```python
from build123d import *

# Parameters (mm, degrees)
CIRPATTERN1_COUNT = 8


with BuildPart() as part:
    # Sketch1 → Revolve2 (revolve)
    with BuildSketch(Plane.XY, mode=Mode.PRIVATE) as revolve2_sk:
        with BuildLine():
            Line((71.638455479, 109.927347077), (76.2, 109.927347077))
            Line((76.2, 109.927347077), (76.2, -212.12767375))
            Line((76.2, -212.12767375), (53.792460136, -212.12767375))
            Line((53.792460136, -212.12767375), (53.792460136, -59.72767375))
            add(Edge.make_bspline(
                [(53.792460136, -59.72767375), (53.792458904, -59.65714368), (53.79192976, -59.515566627), (53.789553906, -59.18172514), (53.783229304, -58.904956016), (53.773743812, -58.532728011), (53.761100911, -58.212998146), (53.741350078, -57.781754967), (53.711337732, -57.281120424), (53.667125562, -56.68815869), (53.588220883, -55.848640892), (53.488359283, -55.008326387), (53.367608198, -54.172595959), (53.197743223, -53.17258577), (53.002996576, -52.177603354), (52.777307499, -51.188699619), (52.520946592, -50.207649576), (52.240221697, -49.233238281), (51.935281085, -48.266129768), (51.544470164, -47.149295616), (51.050452679, -45.89056896), (50.509666057, -44.651129364), (49.922993218, -43.432862093), (49.291052508, -42.237253813), (48.615057493, -41.066315461), (47.895407771, -39.921133247), (47.134034376, -38.804236838), (46.430801288, -37.851612392), (45.804470156, -37.055832736), (45.263749892, -36.403541902), (44.826059154, -35.894408258), (44.42570839, -35.447153287), (44.092389699, -35.084791818), (43.784856817, -34.760500788), (43.585004597, -34.55171009), (43.35532426, -34.318676929), (43.254715338, -34.217322698), (43.20484319, -34.167450311)],
                knots=[0.082637729, 0.082637729, 0.082637729, 0.082637729, 0.082637729, 0.092574926, 0.102512123, 0.11244932, 0.122386517, 0.132323714, 0.142260911, 0.162135305, 0.182009699, 0.201884093, 0.24163288, 0.261507274, 0.281381668, 0.321130456, 0.360879243, 0.380753637, 0.400628031, 0.440376819, 0.480125606, 0.519874394, 0.559623181, 0.599371969, 0.639120757, 0.678869544, 0.718618332, 0.75836712, 0.798115907, 0.817990301, 0.837864695, 0.857739089, 0.877613483, 0.88755068, 0.897487877, 0.907425074, 0.91736227, 0.91736227, 0.91736227, 0.91736227, 0.91736227], degree=4))
            Line((43.20484319, -34.167450311), (34.597214993, -25.559822115))
            add(Edge.make_bspline(
                [(24.01, 0), (24.010001231, -0.070528647), (24.010530378, -0.21358419), (24.012906064, -0.543182916), (24.019230459, -0.824160397), (24.028715581, -1.194822072), (24.041357874, -1.513435058), (24.057158099, -1.861939603), (24.076113358, -2.193706872), (24.103750973, -2.6180694), (24.143219181, -3.122033947), (24.214231843, -3.879978675), (24.334058816, -4.886450388), (24.510418185, -6.05671076), (24.761817377, -7.385166415), (25.062727461, -8.703574514), (25.412702774, -10.009637208), (25.811293137, -11.301819596), (26.257877549, -12.578099334), (26.751935483, -13.836887483), (27.292605285, -15.076197128), (27.879411553, -16.294609793), (28.511071567, -17.489938793), (29.187464568, -18.661287756), (29.906377277, -19.805743395), (30.668954178, -20.923860073), (31.370099373, -21.874411759), (31.999668305, -22.673445479), (32.535060601, -23.320422136), (32.983187953, -23.840005015), (33.419382213, -24.329816244), (33.846758309, -24.788484388), (34.156490828, -25.113868308), (34.447792147, -25.409649045), (34.547344615, -25.50994993), (34.597214993, -25.559822115)],
                knots=[0.082637729, 0.082637729, 0.082637729, 0.082637729, 0.082637729, 0.092574926, 0.102512123, 0.11244932, 0.122386517, 0.132323714, 0.142260911, 0.152198108, 0.162135305, 0.182009699, 0.201884093, 0.24163288, 0.281381668, 0.321130456, 0.360879243, 0.400628031, 0.440376819, 0.480125606, 0.519874394, 0.559623181, 0.599371969, 0.639120757, 0.678869544, 0.718618332, 0.75836712, 0.798115907, 0.817990301, 0.837864695, 0.857739089, 0.877613483, 0.897487877, 0.907425074, 0.91736227, 0.91736227, 0.91736227, 0.91736227, 0.91736227], degree=4))
            add(Edge.make_bspline(
                [(24.01, 0), (24.010000626, 0.035892652), (24.010538457, 0.11011369), (24.012955849, 0.267641069), (24.019393694, 0.427064117), (24.031465725, 0.646764266), (24.052367213, 0.901433328), (24.086116845, 1.202537273), (24.137431431, 1.542050498), (24.201475827, 1.880996777), (24.278073727, 2.21635442), (24.367255697, 2.549239421), (24.468673539, 2.878092645), (24.582551197, 3.203347041), (24.708128897, 3.523627157), (24.846218103, 3.839666733), (24.995002427, 4.149282184), (25.156944348, 4.454783123), (25.327420631, 4.751301575), (25.513446847, 5.045703861), (25.702720396, 5.325518936), (25.9153376, 5.610727543), (26.0898085, 5.832913647), (26.277277882, 6.049951637), (26.415487374, 6.208641646), (26.581374196, 6.382121779), (26.655452387, 6.458478841), (26.706211329, 6.50923965)],
                knots=[0.082568816, 0.082568816, 0.082568816, 0.082568816, 0.082568816, 0.102426634, 0.122284453, 0.142142271, 0.162000089, 0.201715725, 0.241431362, 0.281146998, 0.320862634, 0.360578271, 0.400293907, 0.440009544, 0.47972518, 0.519440816, 0.559156453, 0.598872089, 0.638587725, 0.678303362, 0.718018998, 0.757734635, 0.797450271, 0.837165907, 0.857023726, 0.876881544, 0.91659718, 0.91659718, 0.91659718, 0.91659718, 0.91659718], degree=4))
            add(Edge.make_bspline(
                [(26.706211329, 6.50923965), (49.172333461, 34.635954224), (71.638455479, 109.927347077)],
                knots=[0, 0, 0, 1, 1, 1], degree=2))
        make_face()
    revolve(revolve2_sk.sketch.rotate(Axis((0, 0, 0), (0, -1, 0)), 90), axis=Axis((0, 0, 0), (0, -1, 0)))

    # Sketch4 → 3_8-24 Tapped Hole1 (revolve, cut)
    with BuildSketch(Plane(origin=(66.675, -212.12767375, 0), x_dir=(0, 0, -1), z_dir=(1, 0, 0))):
        Polygon((0, 0), (0, 27.534688714), (4.2164, 25.00122), (4.2164, 0), align=None)
    f_3_8_24_tapped_hole1 = revolve(axis=Axis((66.675, -218.47767375, 0), (0, 1, 0)), mode=Mode.SUBTRACT)

    # CirPattern1: 3_8-24 Tapped Hole1 ×8 about axis
    cirpattern1_axis = Axis((0, 0, 0), (0, 1, 0))
    for i in range(1, CIRPATTERN1_COUNT):
        add(f_3_8_24_tapped_hole1.rotate(cirpattern1_axis, i * 360 / CIRPATTERN1_COUNT), mode=Mode.SUBTRACT)


solid = part.part
```
Work out the finished part from the listing and answer in its coordinate system (mm). A direction names the side the tool comes from. Coordinates: 2 decimals unless noted, no trailing zeros. Order: outer loops, then holes, each group sorted by start corner. A loop starts at its lowest first (then second) coordinate and runs counter-clockwise, first axis right, second up. Notation, with made-up numbers: M -33.5,41.25 L -6.5,41.25 A24 ccw -6.5,69.25 Z; hole C 61,38.25 d4. An arc over 180 degrees is marked long. Use CSV: the item, a comma, the result in double quotes.
1) Determine the mould class of faces 1 (the face through (74.388, -53.355, -16.519)), 2 (the face through (56, 109.927, -45)), 3 (the face through (-34.72, -25.98, -4.56)) for opening direction X: released by +X, released by -X, zero draft, split by the parting line, or undercut.
Worked out:
face 1,"split by the parting line"
face 2,"zero draft"
face 3,"undercut"
2) For faces 4 (the face through (47.329, -199.802, -42.934)), 5 (the face through (-51.2, -212.128, -17.3)), determine the directions among +Z, -Z, +X, -X, +Y, -Y from which every point of the face is accessible in a straight line to the end or side of a thin tool.
Worked out:
face 4,"-Y"
face 5,"+Z, -Z, +X, -X, -Y"
3) Section A-A on y = -104 is taken. Write down the section's boundary in (x, z), plus the area to 3 significant figures.
Worked out:
outline,"C 0,0 d152.4; hole C 0,0 d107.58"
area,"9,150 mm^2"
4) Flat-ended cylindrical pins translate along their axes: pin 1 Ø12 at (x, z) = (43, -5.5) entering from +Y; pin 2 Ø5 at (x, z) = (0, 66.675) entering from -Y; pin 3 Ø11 at (x, z) = (-66.675, 0) entering from -Y; pin 4 Ø1 at (y, z) = (35, 26) entering from -X. Find the tip coordinate at first contact, or state that the pin passes through.
Worked out:
pin 1,"stops at y = 46.84"
pin 2,"stops at y = -186.1"
pin 3,"stops at y = -212.13"
pin 4,"stops at x = -71.81"
5) Consider line 1 (Z direction, x = -2, y = -118.5); line 2 (X direction, y = -170, z = -48); line 3 (X direction, y = 89.5, z = -19). Determine where each line is inside the solid, lowest interval first. Write a range as [from, to].
Worked out:
line 1,"z = [-76.17, -53.76], [53.76, 76.17]"
line 2,"x = [-59.18, -24.28], [24.28, 59.18]"
line 3,"x = [-73.79, -62.43], [62.43, 73.79]"
